CAD build for the part. Positions are in the model's coordinates, mm. A direction names the side the tool comes from. Round coordinates to 2 decimals unless told otherwise and drop trailing zeros. Loops run counter-clockwise (first coordinate to the right, second up) from the corner with the lowest first, then second, coordinate; pieces in that order, holes last. Notation, with made-up numbers: M 75.5,63.5 L 80.5,63.5 A27 ccw 80.5,94.5 Z; hole C 37.5,30 d10. An arc over 180 degrees is marked long. Use a Markdown table: item, result. Add a question column.
(1) Band-saw the part on B-B, the plane z = 2.3. Write the cut outline in (x, y).
(2) Band-saw the part on A-A, the plane x = 2.75. Write the cut outline in (y, z), and give its area (3 significant figures).
(3) Flat gauge pins, fed straight in: P1, Ø1.5, axis at x = -4, z = 3, coming from the -Y side; P2, Ø2, axis at x = -0.5, z = 2.5, coming from the -Y side; P3, Ø0.8, axis at y = 0, z = 3, coming from the -X side; P4, Ø0.9, axis at y = 0, z = 3, coming from the +X side. Where does each tip first touch, or does it go through?
(4) Wall check: L1, parallel to X at y = 0.25, z = 3.7; L2, parallel to Y at x = 0.5, z = 0.8; L3, parallel to X at y = 1.25, z = 3.45. Give the ranges that are in metal, low to high.
(5) Band-saw the part on C-C, the plane x = 0.5. Write the cut outline in (y, z), and give its area (3 significant figures).
(6) Band-saw the part on D-D, the plane y = 3. Write the cut outline in (x, z), and give its area (3 significant figures).
(7) Which spindle directions (+Z, -Z, +X, -X, +Y, -Y) get a long thin tool onto all of the face, cutting with end or side? Do faces 1 (the face through (0, 2, 3)), 2 (the face through (0, -2, 3)), 3 (the face through (-1.25, 0, 2)), 4 (the face through (-5, 1.5, 3)), 5 (the face through (-5, -1.5, 3)). Say none if no direction does.
(8) Two-plate mould, pull along X, no slides. Class faces 6 (the face through (1.25, 0, 2)), 7 (the face through (0, -3.5, 1)), 8 (the face through (-8, 0, 3)): released by +X, released by -X, zero draft, split by the parting line, or undercut.
from build123d import *

# Parameters (mm, degrees)
BOX001_W       = 2.5
BOX001_H       = 1.5
BOX001_DEPTH   = 10
BOX_W          = 16
BOX_H          = 3
BOX_DEPTH      = 5
CYLINDER_R     = 2
CYLINDER_DEPTH = 5
BOX002_W       = 20
BOX002_H       = 7
BOX002_DEPTH   = 2


with BuildPart() as cube001:
    # Box001 → Box001 (new body)
    with BuildSketch(Plane(origin=(-1.25, -0.75, 0), x_dir=(1, 0, 0), z_dir=(0, 0, 1))):
        with Locations((1.25, 0.75)):
            Rectangle(BOX001_W, BOX001_H)
    extrude(amount=BOX001_DEPTH)


with BuildPart() as cube:
    # Box → Box (new body)
    with BuildSketch(Plane(origin=(-8, -1.5, 0), x_dir=(1, 0, 0), z_dir=(0, 0, 1))):
        with Locations((8, 1.5)):
            Rectangle(BOX_W, BOX_H)
    extrude(amount=BOX_DEPTH)


with BuildPart() as fusion:
    # Cylinder → Cylinder (new body)
    with BuildSketch(Plane.XY):
        Circle(CYLINDER_R)
    extrude(amount=CYLINDER_DEPTH)

    # Fusion: union Cube
    add(cube.part)


with BuildPart() as cut:
    # Box002 → Box002 (new body)
    with BuildSketch(Plane(origin=(-10, -3.5, 0), x_dir=(1, 0, 0), z_dir=(0, 0, 1))):
        with Locations((10, 3.5)):
            Rectangle(BOX002_W, BOX002_H)
    extrude(amount=BOX002_DEPTH)

    # Fusion001: union Fusion
    add(fusion.part)

    # Cut: cut Cube001
    add(cube001.part, mode=Mode.SUBTRACT)


solid = cut.part
Return value:
| question | item | result |
|---|---|---|
| 1 | outline | M -8,-1.5 L -1.32,-1.5 A2 ccw 1.32,-1.5 L 8,-1.5 L 8,1.5 L 1.32,1.5 A2 ccw -1.32,1.5 L -8,1.5 Z; hole M -1.25,-0.75 L 1.25,-0.75 L 1.25,0.75 L -1.25,0.75 Z |
| 2 | outline | M -3.5,0 L 3.5,0 L 3.5,2 L 1.5,2 L 1.5,5 L -1.5,5 L -1.5,2 L -3.5,2 Z |
| 2 | area | 23.0 mm^2 |
| 3 | P1 | y = -1.5 |
| 3 | P2 | y = -3.5 |
| 3 | P3 | x = -8 |
| 3 | P4 | x = 8 |
| 4 | L1 | -8 to -1.25, 1.25 to 8 |
| 4 | L2 | -3.5 to -0.75, 0.75 to 3.5 |
| 4 | L3 | -8 to 8 |
| 5 | outline | M -3.5,0 L -0.75,0 L -0.75,5 L -1.94,5 L -1.94,2 L -3.5,2 Z; M 0.75,0 L 3.5,0 L 3.5,2 L 1.94,2 L 1.94,5 L 0.75,5 Z |
| 5 | area | 18.1 mm^2 |
| 6 | outline | M -10,0 L 10,0 L 10,2 L -10,2 Z |
| 6 | area | 40.0 mm^2 |
| 7 | face 1 | +Z, +Y |
| 7 | face 2 | +Z, -Y |
| 7 | face 3 | +Z, -Z |
| 7 | face 4 | +Z, -X, +Y |
| 7 | face 5 | +Z, -X, -Y |
| 8 | face 6 | undercut |
| 8 | face 7 | zero draft |
| 8 | face 8 | released by -X |
